For this review, take the finished solid that the model builds, in its own axes (mm). A direction names the side the tool comes from. Give positions to 0.01 mm unless a question says otherwise; leave off trailing zeros. Write each loop counter-clockwise with the first axis right and the second up, starting at its lowest first coordinate (ties: lowest second). Pieces come first, ordered by that corner, then holes.
1) Wall thickness on line 1 along Z through (x, y) = (20, 3); line 2 along Y through (x, z) = (-5, 7); line 3 along Z through (x, y) = (20.25, 4.7): over which ranges is each line inside the solid? List them lowest first.
2) We need section B-B on y = 32.5. Give the boundary of the cut face in (x, z), and give its area (3 significant figures).
3) Draft analysis for pull direction Y (two halves, no side actions). For faces 1 (the face through (0, 87, 0)), 2 (the face through (-4.8, 32.9, 8.2)), 3 (the face through (-0.1, 29, 6.2)), 4 (the face through (0.02, 61.4, -9.85)), state which applies: pulls with the +Y half, pulls with the -Y half, needs draft (parallel to the pull), parting line crosses it, or undercut.
4) We need section A-A on x = 20.25. Give the boundary of the cut face in (y, z).
5) Machinability: for faces 5 (the face through (11, 6, 11)), 6 (the face through (2, 20, 9)), 7 (the face through (0.02, 29.21, -9.86)), 8 (the face through (-8.519, 61.402, -4.946)), which of the approach directions +Z, -Z, +X, -X, +Y, -Y give a long, thin tool a straight path to every point of the face, cutting with its end or side? Answer none if there is none.
6) We need section C-C on z = 17.5. Give the boundary of the cut face in (x, y), and give its area (3 significant figures).
7) For P1, Ø5, axis at x = -6, y = 62, coming from the -Z side; P2, Ø1.5, axis at y = 11, z = 12.5, coming from the +X side; P3, Ø12, axis at y = 13.5, z = -4, coming from the +X side, all flat-tipped, find the tip position at first contact; note any pin that passes through.
from build123d import *

# Parameters (mm, degrees)
EXTRUDE_1_DEPTH     = 8
EXTRUDE_2_DEPTH     = 10
SKETCH_5_R          = 3.25
CUT_EXTRUDE_1_DEPTH = 7


with BuildPart() as part:
    # Эскиз1 → Повернуть1 (revolve)
    with BuildSketch(Plane.XY, mode=Mode.PRIVATE) as revolve_1_sk:
        Polygon((0, 0), (-25, 0), (-25, 6), (-15, 6), (-11, 20), (-9, 20), (-9, 22), (-6, 25), (-6, 29), (-6, 37), (-6, 85.4), (-4.4, 87), (0, 87), align=None)
    revolve(revolve_1_sk.sketch.rotate(Axis((0, 0, 0), (0, 1, 0)), 180), axis=Axis((0, 0, 0), (0, 1, 0)))  # turned: the seam where the file's is

    # Эскиз2 → Бобышка-Вытянуть1 (add)
    with BuildSketch(Plane(origin=(0, 29, 0), x_dir=(1, 0, 0), z_dir=(0, 1, 0))):
        Polygon((0, 10.969655115), (-9.5, 5.484827557), (-9.5, -5.484827557), (0, -10.969655115), (9.5, -5.484827557), (9.5, 5.484827557), align=None)
    extrude(amount=EXTRUDE_1_DEPTH)

    # Эскиз3 → Бобышка-Вытянуть2 (add)
    with BuildSketch(Plane(origin=(0, 61.2, 0), x_dir=(1, 0, 0), z_dir=(0, 1, 0))):
        Polygon((9.5, 5.484827557), (0, 10.969655115), (-9.5, 5.484827557), (-9.5, -5.484827557), (0, -10.969655115), (9.5, -5.484827557), align=None)
    extrude(amount=EXTRUDE_2_DEPTH)

    # Эскиз4 → Вырез-Повернуть2 (revolve, cut)
    with BuildSketch(Plane.XY, mode=Mode.PRIVATE) as cut_revolve_2_sk:
        Polygon((-18.160254038, 71.2), (-9.5, 71.2), (-18.160254038, 66.2), align=None)
        Polygon((-18.160254038, 61.2), (-18.160254038, 66.2), (-9.5, 61.2), align=None)
        Polygon((-16.42820323, 37), (-16.42820323, 33), (-9.5, 37), align=None)
        Polygon((-16.42820323, 33), (-16.42820323, 29), (-9.5, 29), align=None)
    revolve(cut_revolve_2_sk.sketch.rotate(Axis((0, 87, 0), (0, 1, 0)), 180), axis=Axis((0, 87, 0), (0, 1, 0)), mode=Mode.SUBTRACT)  # turned: the seam where the file's is

    # Эскиз5 → Вырез-Вытянуть1 (cut, through all)
    with BuildSketch(Plane(origin=(0, 6, 0), x_dir=(1, 0, 0), z_dir=(0, 1, 0))):
        with Locations(Location((-20.25, 0, 0), (0, 0, 180))):  # turned: the seam where the file's is
            Circle(SKETCH_5_R)
        with Locations(Location((20.25, 0, 0), (0, 0, 180))):  # turned: the seam where the file's is
            Circle(SKETCH_5_R)
    extrude(amount=-CUT_EXTRUDE_1_DEPTH, mode=Mode.SUBTRACT)


solid = part.part
Results list:
1. line 1: z = -15 to -3.24, 3.24 to 15
1. line 2: y = 0 to 22.4, 29 to 37, 61.2 to 71.2
1. line 3: z = -14.66 to -3.25, 3.25 to 14.66
2. outline: (-9.5, -5.48) - (0, -10.97) - (9.5, -5.48) - (9.5, 5.48) - (0, 10.97) - (-9.5, 5.48) - close
2. area: 313 mm2
3. face 1: pulls with the +Y half
3. face 2: needs draft
3. face 3: undercut
3. face 4: undercut
4. outline: (0, -14.66) - (6, -14.66) - (6, -3.25) - (0, -3.25) - close; (0, 3.25) - (6, 3.25) - (6, 14.66) - (0, 14.66) - close
5. face 5: +Y
5. face 6: none
5. face 7: -Z
5. face 8: -Z, -X
6. outline: (-17.85, 0) - (17.85, 0) - (17.85, 6) - (-17.85, 6) - close
6. area: 214 mm2
7. P1: stops at z = -8.95
7. P2: stops at x = 6.86
7. P3: stops at x = 14.34
